Here's how the part is built. I have some questions about the finished solid (model axes, mm). Face numbers are marked on the shaded views. A direction names the side the tool comes from. Give positions to 0.01 mm unless a question says otherwise; leave off trailing zeros. Order: outer loops, then holes, each group sorted by start corner. A loop starts at its lowest first (then second) coordinate and runs counter-clockwise, first axis right, second up.
from build123d import *

# Parameters (mm, degrees)
SKETCH1_W               = 76.2
SKETCH1_H               = 50.8
SKETCH1_W_2             = 69.85
SKETCH1_H_2             = 44.45
BOSS_EXTRUDE1_DEPTH     = 173.75
CUT_EXTRUDE1_DEPTH      = 180.682588194
CUT_EXTRUDE1_DEPTH_BACK = 180.682588194
SKETCH2_R               = 5
FILLET1_R               = 6.35


with BuildPart() as part:
    # Sketch1 → Boss-Extrude1 (new body)
    with BuildSketch(Plane.XY):
        Rectangle(SKETCH1_W, SKETCH1_H)
        Rectangle(SKETCH1_W_2, SKETCH1_H_2, mode=Mode.SUBTRACT)
    extrude(amount=BOSS_EXTRUDE1_DEPTH)

    # Sketch2 → Cut-Extrude1 (cut, two sides: drawn at the far end of the back side and taken through both)
    with BuildSketch(Plane(origin=(0, 0, 0), x_dir=(0, 0, -1), z_dir=(1, 0, 0)).offset(-CUT_EXTRUDE1_DEPTH_BACK)):
        with Locations((-165.625, 13.275)):
            Circle(SKETCH2_R)
        with Locations((-8.125, 13.275)):
            Circle(SKETCH2_R)
        Polygon((-173.75, 25.4), (0, 25.4), (0, 21.4), (-31.875, 21.4), (-53.088203436, 0.186796564), (-86.875, 0), (-120.661796564, 0.186796564), (-141.875, 21.4), (-173.75, 21.4), align=None)
    extrude(amount=CUT_EXTRUDE1_DEPTH + CUT_EXTRUDE1_DEPTH_BACK, mode=Mode.SUBTRACT)

    # Fillet1
    fillet1_edges = [part.edges().sort_by_distance(p)[0] for p in [
        (-36.5125, 0.186796564, 53.088203436),
        (-36.5125, 0.186796564, 120.661796564),
        (36.5125, 0.186796564, 53.088203436),
        (36.5125, 0.186796564, 120.661796564),
    ]]
    fillet(fillet1_edges, radius=FILLET1_R)


solid = part.part
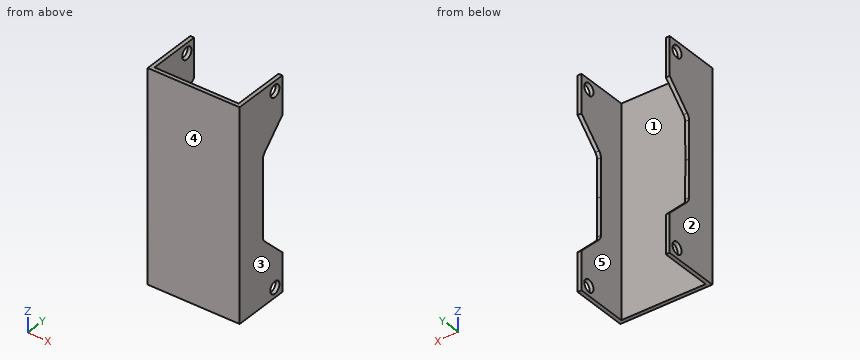
Q1. If we section it at C-C on x = 20: List the corners of the cut face in (y, z) for me (3 decimals).
Filled sheet:
outline: (-25.4, 0) - (-22.225, 0) - (-22.225, 173.75) - (-25.4, 173.75) - close
Q2. For the marked faces 1 and 2, which set-ups out of +Z, -Z, +X, -X, +Y, -Y let a thin tool reach every point of the face, with its end or its side?
Filled sheet:
face 1: +Z, -Z, +Y
face 2: +Z, -Z, -X, +Y, -Y
Q3. If we section it at B-B on z = 19: List the corners of the cut face in (x, y) for me (3 decimals), plus the area to 3 significant figures.
Filled sheet:
outline: (-38.1, -25.4) - (38.1, -25.4) - (38.1, 21.4) - (34.925, 21.4) - (34.925, -22.225) - (-34.925, -22.225) - (-34.925, 21.4) - (-38.1, 21.4) - close
area: 519 mm2
Q4. I need wall thicknesses on L1, parallel to X at y = 0, z = 75.5 (3 decimals); L2, parallel to Y at x = -35, z = 165.5; L3, parallel to Y at x = -14.5, z = 64.5 (3 decimals). Which ranges of each line are inside material? Lowest first, please.
Filled sheet:
L1: x = -38.1 to -34.925, 34.925 to 38.1
L2: y = -25.4 to 8.28, 18.27 to 21.4
L3: y = -25.4 to -22.225
Q5. Thinking about a two-plate mould opening in X: for the marked faces 3, 4 and 5, which applies, released by +X, released by -X, zero draft, split by the parting line, or undercut?
Filled sheet:
face 3: released by +X
face 4: zero draft
face 5: undercut
Q6. I'm going to push a flat-ended pin straight in: P1, Ø1.5, axis at x = -26.5, z = 144.5, coming from the +Y side (3 decimals). Where does the tip first touch, or does it pass through?
Filled sheet:
P1: stops at y = -22.225
Q7. If we section it at D-D on z = 137.5: List the corners of the cut face in (x, y) for me (3 decimals), plus the area to 3 significant figures.
Filled sheet:
outline: (-38.1, -25.4) - (38.1, -25.4) - (38.1, 17.025) - (34.925, 17.025) - (34.925, -22.225) - (-34.925, -22.225) - (-34.925, 17.025) - (-38.1, 17.025) - close
area: 491 mm2
Q8. If we section it at A-A on y = -5: List the corners of the cut face in (x, z) for me (3 decimals), plus the area to 3 significant figures.
Filled sheet:
outline: (-38.1, 0) - (-34.925, 0) - (-34.925, 173.75) - (-38.1, 173.75) - close; (34.925, 0) - (38.1, 0) - (38.1, 173.75) - (34.925, 173.75) - close
area: 1,100 mm2
